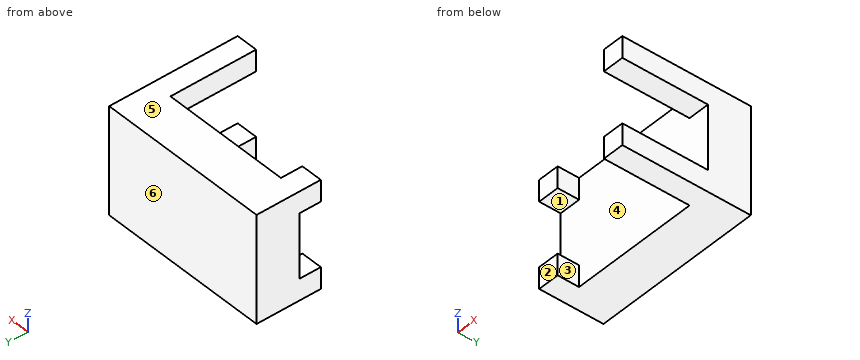
from build123d import *

# Parameters (mm, degrees)
F0_W     = 101.6
F0_H     = 63.5
F1_DEPTH = 25.4
F2_W     = 12.7
F2_H     = 12.7
F3_DEPTH = 12.7
F4_DEPTH = 50.8


with BuildPart() as f1:
    # F0 (on Front) → F1 (new body)
    with BuildSketch(Plane.XZ):
        Rectangle(F0_W, F0_H)
    extrude(amount=F1_DEPTH)

    # F2 (on face) → F3 (join)
    with BuildSketch(Plane.XZ.offset(25.4)):
        with Locations((-44.45, 25.4)):
            Rectangle(F2_W, F2_H)
        with Locations((-44.45, -25.4)):
            Rectangle(F2_W, F2_H)
    extrude(amount=F3_DEPTH)

    # F2 (on face) → F4 (join)
    with BuildSketch(Plane.XZ.offset(25.4)):
        with Locations((44.45, 25.4)):
            Rectangle(F2_W, F2_H)
        with Locations((44.45, -25.4)):
            Rectangle(F2_W, F2_H)
    extrude(amount=F4_DEPTH)


solid = f1.part
The model under review builds one solid part; all positions refer to its coordinate system, in mm. Face numbers are marked on the shaded views. A direction names the side the tool comes from. Give positions to 0.01 mm unless a question says otherwise; leave off trailing zeros. Order: outer loops, then holes, each group sorted by start corner. A loop starts at its lowest first (then second) coordinate and runs counter-clockwise, first axis right, second up. Notation, with made-up numbers: M 84,23.5 L 114,23.5 A24 ccw 114,55.5 Z; hole C 60.5,-12.5 d1. An arc over 180 degrees is marked long. Answer in a Markdown table with one row per item. Add a question column.
1. Add section D-D on z = 26. State the section outline as (x, y) points, plus the area to 3 significant figures.
2. For pin 1 Ø14 at (y, z) = (-57.5, -25.5) entering from -X; pin 2 Ø1 at (x, y) = (-23.5, -27.5) entering from +Z; pin 3 Ø6.5 at (x, z) = (-42, -24.5) entering from -Y; pin 4 Ø1 at (x, z) = (-11, 24.5) entering from -Y, all flat-tipped, find the tip position at first contact; note any pin that passes through.
3. To check wall thickness, follow line 1 along X through (y, z) = (-26, 26); line 2 along Z through (x, y) = (45.5, -42.5); line 3 along X through (y, z) = (-41, -22.5). State the ranges of each line that lie inside material, in increasing order.
4. Add section A-A on y = -32. State the section outline as (x, z) points, plus the area to 3 significant figures.
5. Mouldability with a two-part tool opening along Z and no side actions: class the marked faces 4, 5 and 6 as released by +Z, released by -Z, zero draft, split by the parting line, or undercut.
6. Add section C-C on y = -69.5. State the section outline as (x, z) points, plus the area to 3 significant figures.
7. Machinability: for the marked faces 1, 2 and 3, which of the approach directions +Z, -Z, +X, -X, +Y, -Y give a long, thin tool a straight path to every point of the face, cutting with its end or side? Answer none if there is none.
8. Add section B-B on x = -41. State the section outline as (y, z) points, plus the area to 3 significant figures.
The answers:
| question | item | result |
|---|---|---|
| 1 | outline | M -50.8,-38.1 L -38.1,-38.1 L -38.1,-25.4 L 38.1,-25.4 L 38.1,-76.2 L 50.8,-76.2 L 50.8,0 L -50.8,0 Z |
| 1 | area | 3,390 mm2 |
| 2 | pin 1 | x = 38.1 |
| 2 | pin 2 | through |
| 2 | pin 3 | y = -38.1 |
| 2 | pin 4 | y = -25.4 |
| 3 | line 1 | -50.8 to -38.1, 38.1 to 50.8 |
| 3 | line 2 | -31.75 to -19.05, 19.05 to 31.75 |
| 3 | line 3 | 38.1 to 50.8 |
| 4 | outline | M -50.8,-31.75 L -38.1,-31.75 L -38.1,-19.05 L -50.8,-19.05 Z; M -50.8,19.05 L -38.1,19.05 L -38.1,31.75 L -50.8,31.75 Z; M 38.1,-31.75 L 50.8,-31.75 L 50.8,-19.05 L 38.1,-19.05 Z; M 38.1,19.05 L 50.8,19.05 L 50.8,31.75 L 38.1,31.75 Z |
| 4 | area | 645 mm2 |
| 5 | face 4 | undercut |
| 5 | face 5 | released by +Z |
| 5 | face 6 | zero draft |
| 6 | outline | M 38.1,-31.75 L 50.8,-31.75 L 50.8,-19.05 L 38.1,-19.05 Z; M 38.1,19.05 L 50.8,19.05 L 50.8,31.75 L 38.1,31.75 Z |
| 6 | area | 323 mm2 |
| 7 | face 1 | +X, -X, -Y |
| 7 | face 2 | +Z, -Z, -X, -Y |
| 7 | face 3 | +Z, -Z, -Y |
| 8 | outline | M -38.1,-31.75 L 0,-31.75 L 0,31.75 L -38.1,31.75 L -38.1,19.05 L -25.4,19.05 L -25.4,-19.05 L -38.1,-19.05 Z |
| 8 | area | 1,940 mm2 |
